```python
from build123d import *

# Parameters (mm, degrees)
SKETCH2_W                    = 57.15
SKETCH2_H                    = 31.75
BASE_FLANGE1_DEPTH           = 3.175
EDGE_FLANGE1_STRIP_W         = 14.7
EDGE_FLANGE1_STRIP_H         = 3.175
EDGE_FLANGE1_STRIP_CUT_DEPTH = 31.75
EDGE_FLANGE1_DEPTH           = 31.75
CUT_EXTRUDE1_DEPTH           = 77.59584682
CUT_EXTRUDE1_DEPTH_BACK      = 3.175
M6_CLEARANCE_HOLE1_D         = 6.6


# Sheet-metal steps are written as plain solids
with BuildPart() as part:
    # Sketch2 → Base-Flange1 (new body)
    with BuildSketch(Plane.XY):
        Rectangle(SKETCH2_W, SKETCH2_H)
    extrude(amount=BASE_FLANGE1_DEPTH)

    # Edge-Flange1 strip (across the edge) → Edge-Flange1 strip cut (cut)
    with BuildSketch(Plane(origin=(28.575, -15.875, 3.175), x_dir=(-1, 0, 0), z_dir=(0, 1, 0))):
        with Locations((-6.35, -1.5875)):
            Rectangle(EDGE_FLANGE1_STRIP_W, EDGE_FLANGE1_STRIP_H)
    extrude(amount=EDGE_FLANGE1_STRIP_CUT_DEPTH, mode=Mode.SUBTRACT)

    # Edge-Flange1 section (across the edge) → Edge-Flange1 (add)
    with BuildSketch(Plane(origin=(28.575, -15.875, 3.175), x_dir=(-1, 0, 0), z_dir=(0, 1, 0))):
        with BuildLine():
            Line((-3.175, 1), (-3.175, 41.275))
            Line((-3.175, 41.275), (0, 41.275))
            Line((0, 41.275), (0, 1))
            ThreePointArc((0, 1), (0.292893219, 0.292893219), (1, 0))
            Line((1, 0), (1, -3.175))
            ThreePointArc((1, -3.175), (-1.952170811, -1.952170811), (-3.175, 1))
        make_face()
    extrude(amount=EDGE_FLANGE1_DEPTH)

    # Sketch10 → Cut-Extrude1 (cut, two sides: drawn at the far end of the back side and taken through both)
    with BuildSketch(Plane(origin=(31.75, 0, 0), x_dir=(0, 0, -1), z_dir=(1, 0, 0)).offset(-CUT_EXTRUDE1_DEPTH_BACK)):
        Polygon((-4.175, 15.875), (-44.45, -15.875), (-44.45, 15.875), align=None)
    extrude(amount=CUT_EXTRUDE1_DEPTH + CUT_EXTRUDE1_DEPTH_BACK, mode=Mode.SUBTRACT)

    # M6 Clearance Hole1 (through all)
    with Locations(Plane.XY.offset(3.175)):
        with Locations((0, 0)):
            Hole(M6_CLEARANCE_HOLE1_D / 2)


solid = part.part
```
Geometry check sheet. Reference: the model listing, model coordinates, mm. A direction names the side the tool comes from. Coordinates: 2 decimals unless noted, no trailing zeros. Loops run counter-clockwise (first coordinate to the right, second up) from the corner with the lowest first, then second, coordinate; pieces in that order, holes last. Notation, with made-up numbers: (15.5, 40) - (20.5, 40) arc R32 ccw to (20.5, 77) - close; hole circle Ø8 at (9.25, -17.5). An arc over 180 degrees is marked (long way). One line per item, written item: value. Start each with the question number.
(1) Material ranges on line 1 (Y direction, x = 0, z = 1) (3 decimals); line 2 (Z direction, x = 20, y = 13) (3 decimals); line 3 (X direction, y = 6.5, z = 15) (3 decimals), recorded low to high. Write a range as [from, to].
(2) Cross-section at A-A on x = 0. Enter the section's corners in (y, z) (3 decimals), plus the area to 3 significant figures.
(3) Cross-section at D-D on x = -23.5. Enter the section's corners in (y, z) (3 decimals), plus the area to 3 significant figures.
(4) Cross-section at C-C on y = 12. Enter the section's corners in (x, z) (3 decimals).
(5) Cross-section at B-B on y = 1.5. Enter the section's corners in (x, z) (3 decimals), plus the area to 3 significant figures.
(6) Depth check by flat-ended pin: P1, Ø10, axis at y = -1.5, z = 27.5, coming from the -X side (3 decimals); P2, Ø1, axis at x = 7.5, y = 6, coming from the +Z side (3 decimals); P3, Ø6, axis at x = 22.5, z = 9, coming from the +Y side. Enter the tip coordinate at first touch or a pass-through.
(7) Mould release check, pull along X, two halves, no side actions. Record for faces 3 (the cylindrical face through (2.43, 2.23, 1.57)), 4 (the cylindrical face through (30.495, -0.222, 1.191)), 5 (the flat face through (30.14, 0.222, 24.031)): released by +X, released by -X, zero draft, split by the parting line, or undercut.
(8) Tool access check on faces 1 (the flat face through (-1, 4, 3.175)), 2 (the flat face through (1, 15.875, 2)). Record the directions out of +Z, -Z, +X, -X, +Y, -Y that give a thin tool (end or side, any length) a straight path to the whole face; none if there is none.
Results below:
1. line 1: y = [-15.875, -3.3], [3.3, 15.875]
1. line 2: z = [0, 3.175]
1. line 3: x = [28.575, 31.75]
2. outline: (-15.875, 0) - (-3.3, 0) - (-3.3, 3.175) - (-15.875, 3.175) - close; (3.3, 0) - (15.875, 0) - (15.875, 3.175) - (3.3, 3.175) - close
2. area: 79.9 mm2
3. outline: (-15.875, 0) - (15.875, 0) - (15.875, 3.175) - (-15.875, 3.175) - close
3. area: 101 mm2
4. outline: (-28.575, 0) - (27.575, 0) arc R4.175 ccw to (31.75, 4.175) - (31.75, 9.09) - (28.575, 9.09) - (28.575, 4.175) arc R1 cw to (27.575, 3.175) - (-28.575, 3.175) - close
5. outline: (-28.575, 0) - (-2.939, 0) - (-2.939, 3.175) - (-28.575, 3.175) - close; (2.939, 0) - (27.575, 0) arc R4.175 ccw to (31.75, 4.175) - (31.75, 22.41) - (28.575, 22.41) - (28.575, 4.175) arc R1 cw to (27.575, 3.175) - (2.939, 3.175) - close
5. area: 230 mm2
6. P1: stops at x = 28.575
6. P2: stops at z = 3.175
6. P3: passes through
7. face 3: undercut
7. face 4: released by +X
7. face 5: zero draft
8. face 1: +Z, -X, +Y, -Y
8. face 2: +Z, -Z, +X, -X, +Y
